The model under review builds one solid part; all positions refer to its coordinate system, in mm. A direction names the side the tool comes from. Coordinates: 2 decimals unless noted, no trailing zeros. Write each loop counter-clockwise with the first axis right and the second up, starting at its lowest first coordinate (ties: lowest second). Pieces come first, ordered by that corner, then holes.
1) Add section B-B, the plane y = -1.65. State the section outline as (x, z) points.
2) Add section C-C, the plane y = 0. State the section outline as (x, z) points.
3) Machinability: for faces 1 (the cylindrical face through (0.945, 0.724, 0.178)), 2 (the cylindrical face through (2.46, -0.11, 12.99)), which of the approach directions +Z, -Z, +X, -X, +Y, -Y give a long, thin tool a straight path to every point of the face, cutting with its end or side? Answer none if there is none.
4) Mouldability with a two-part tool opening along Z and no side actions: class faces 3 (the flat face through (-1, -1, -12.7)), 4 (the cylindrical face through (2.46, -0.11, -12.98)), 5 (the flat face through (1, -1, 12.7)) as released by +Z, released by -Z, zero draft, split by the parting line, or undercut.
5) For P1, Ø1.5, axis at x = 0, y = -1, coming from the -Z side; P2, Ø1, axis at x = -0.5, y = -1, coming from the +Z side; P3, Ø1.5, axis at x = 1, y = -2, coming from the +Z side, all flat-tipped, find the tip position at first contact; note any pin that passes through.
6) Add section D-D, the plane x = 0.7. State the section outline as (y, z) points, then the cut area to 3 significant figures.
7) Add section A-A, the plane x = -1.5. State the section outline as (y, z) points, then the cut area to 3 significant figures.
8) For line 1 (Z direction, x = -1.3, y = 2); line 2 (Z direction, x = 0.65, y = -1.55); line 3 (X direction, y = 0.5, z = -2.75), list the stretches that pass through material, from the lowest coordinate up.
from build123d import *
from OCP.BRepFilletAPI import BRepFilletAPI_MakeChamfer

# Parameters (mm, degrees)
SKETCH1_R           = 1.190625
EXTRUDE1_DEPTH      = 12.7
SKETCH1_W           = 9.8552
SKETCH1_H           = 1.27
EXTRUDE1_2_DEPTH    = 12.7
SKETCH20_R          = 1.4224
EXTRUDE24_DEPTH     = 20.045522232
CHAMFER2_SIZE       = 0.635
CHAMFER2_SIZE2      = 0.551997079
EXTRUDE4_DEPTH      = 19.94700397
EXTRUDE4_DEPTH_BACK = 19.94700397
SKETCH8_W           = 5.6896
SKETCH8_H           = 8.466666666
SKETCH9_R           = 1.190625
EXTRUDE5_DEPTH      = 8.466666667


# Read off the part's stored shape, not the designer's step: Mirror2
with BuildPart() as part:
    # Sketch1 → Extrude1 (new, symmetric)
    with BuildSketch(Plane.XY):
        with BuildLine():
            Line((12.7, -2.157017049), (1.190625, -2.157017049))
            ThreePointArc((1.190625, -2.157017049), (-1.856577095, 1.619701185), (2.298588957, -0.887017049))
            Line((2.298588957, -0.887017049), (12.7, -0.887017049))
            Line((12.7, -0.887017049), (12.7, -2.157017049))
        make_face()
        Circle(SKETCH1_R, mode=Mode.SUBTRACT)
    extrude(amount=EXTRUDE1_DEPTH, both=True)

    # Mirror2 outline → Mirror2 (revolve, cut)
    with BuildSketch(Plane(origin=(8.3312, 0, -7.8486), x_dir=(1, 0, 0), z_dir=(0, 0, 1))):
        Polygon((1.784715731, -0.887017049), (0, -0.887017049), (0, -1.93881362), (1.4224, -1.93881362), (1.4224, -1.30381362), align=None)
    revolve(axis=Axis((8.3312, 0, -7.8486), (0, 1, 0)), mode=Mode.SUBTRACT)

    # Mirror2 2 outline → Mirror2 2 (revolve, cut)
    with BuildSketch(Plane(origin=(8.3312, 0, 7.8486), x_dir=(1, 0, 0), z_dir=(0, 0, 1))):
        Polygon((0, -0.887017049), (0, -1.93881362), (1.4224, -1.93881362), (1.4224, -1.30381362), (1.784715731, -0.887017049), align=None)
    revolve(axis=Axis((8.3312, 0, 7.8486), (0, 1, 0)), mode=Mode.SUBTRACT)

    # Sketch8 → Extrude4 (cut, two sides: drawn at the far end of the back side and taken through both)
    with BuildSketch(Plane(origin=(0, 0, 0), x_dir=(1, 0, 0), z_dir=(0, 1, 0)).offset(-EXTRUDE4_DEPTH_BACK)):
        Rectangle(SKETCH8_W, SKETCH8_H)
    extrude(amount=EXTRUDE4_DEPTH + EXTRUDE4_DEPTH_BACK, mode=Mode.SUBTRACT)


with BuildPart() as body_2:
    # Sketch1 → Extrude1 2 (new, symmetric)
    with BuildSketch(Plane.XY):
        with Locations((-7.7724, -1.30381362)):
            Rectangle(SKETCH1_W, SKETCH1_H)
    extrude(amount=EXTRUDE1_2_DEPTH, both=True)

    # Sketch20 → Extrude24 (cut, through all)
    with BuildSketch(Plane(origin=(0, -0.66881362, 0), x_dir=(1, 0, 0), z_dir=(0, 1, 0))):
        with Locations(Location((-8.3312, 7.8486, 0), (0, 0, 270))):
            Circle(SKETCH20_R)
        with Locations(Location((-8.3312, -7.8486, 0), (0, 0, 270))):
            Circle(SKETCH20_R)
    extrude(amount=-EXTRUDE24_DEPTH, mode=Mode.SUBTRACT)

    # Chamfer2: one chamfer whose edges measure the first distance from different faces: ONE call of the kernel's chamfer builder (chamfer() names one face for all edges)
    chamfer2_edges_1 = [body_2.edges().sort_by_distance(p)[0] for p in [
        (-8.3312, -0.66881362, -9.271),
    ]]
    chamfer2_side_1 = [body_2.faces().sort_by_distance(p)[0] for p in [
        (-8.3312, -1.30381362, -9.271),
    ]]
    chamfer2_edges_2 = [body_2.edges().sort_by_distance(p)[0] for p in [
        (-8.3312, -0.66881362, 6.4262),
    ]]
    chamfer2_side_2 = [body_2.faces().sort_by_distance(p)[0] for p in [
        (-8.3312, -1.30381362, 6.4262),
    ]]
    chamfer2 = BRepFilletAPI_MakeChamfer(body_2.part.solid().wrapped)
    for e in chamfer2_edges_1:
        chamfer2.Add(CHAMFER2_SIZE, CHAMFER2_SIZE2, e.wrapped, chamfer2_side_1[0].wrapped)  # the first distance lies on this face
    for e in chamfer2_edges_2:
        chamfer2.Add(CHAMFER2_SIZE, CHAMFER2_SIZE2, e.wrapped, chamfer2_side_2[0].wrapped)  # the first distance lies on this face
    add(Compound.cast(chamfer2.Shape()), mode=Mode.REPLACE)

    # Sketch9 → Extrude5 (add)
    with BuildSketch(Plane.XY.offset(-4.233333333)):
        with BuildLine():
            Line((-2.371286314, -0.66881362), (-2.8448, -0.66881362))
            Line((-2.8448, -0.66881362), (-2.8448, -1.93881362))
            Line((-2.8448, -1.93881362), (-1.520300032, -1.93881362))
            ThreePointArc((-1.520300032, -1.93881362), (2.046786768, 1.371486189), (-2.371286314, -0.66881362))
        make_face()
        with Locations(Location((0, 0, 0), (0, 0, 180))):
            Circle(SKETCH9_R, mode=Mode.SUBTRACT)
    extrude(amount=EXTRUDE5_DEPTH)


with BuildPart() as body_3:
    # Sketch6 → Revolve1 (revolve)
    with BuildSketch(Plane(origin=(0, 0, 0), x_dir=(1, 0, 0), z_dir=(0, 1, 0))):
        with BuildLine():
            Line((-2.4638, -12.7), (-2.4638, -13.2715))
            ThreePointArc((-2.4638, -13.2715), (-1.264606924, -13.698253184), (0, -13.843))
            Line((0, -13.843), (0, 13.843))
            ThreePointArc((0, 13.843), (-1.264606924, 13.698253184), (-2.4638, 13.2715))
            Line((-2.4638, 13.2715), (-2.4638, 12.7))
            Line((-2.4638, 12.7), (-1.190625, 12.7))
            Line((-1.190625, 12.7), (-1.190625, -12.7))
            Line((-1.190625, -12.7), (-2.4638, -12.7))
        make_face()
    revolve(axis=Axis((0, 0, -13.843), (0, 0, 1)))


solid = body_3.part
Geometry results:
1. outline: (-1.83, -13.27) arc R5.35 ccw to (1.83, -13.27) - (1.83, -12.7) - (-1.83, -12.7) - close; (-1.83, 12.7) - (1.83, 12.7) - (1.83, 13.27) arc R5.35 ccw to (-1.83, 13.27) - close
2. outline: (-2.46, -13.27) arc R5.6 ccw to (2.46, -13.27) - (2.46, -12.7) - (1.19, -12.7) - (1.19, 12.7) - (2.46, 12.7) - (2.46, 13.27) arc R5.6 ccw to (-2.46, 13.27) - (-2.46, 12.7) - (-1.19, 12.7) - (-1.19, -12.7) - (-2.46, -12.7) - close
3. face 1: none
3. face 2: +Z, -Z
4. face 3: undercut
4. face 4: zero draft
4. face 5: undercut
5. P1: stops at z = -13.84
5. P2: stops at z = 13.81
5. P3: stops at z = 13.64
6. outline: (-2.36, -13.27) arc R5.55 ccw to (2.36, -13.27) - (2.36, -12.7) - (0.96, -12.7) - (0.96, 12.7) - (2.36, 12.7) - (2.36, 13.27) arc R5.55 ccw to (-2.36, 13.27) - (-2.36, 12.7) - (-0.96, 12.7) - (-0.96, -12.7) - (-2.36, -12.7) - close
6. area: 57.7 mm2
7. outline: (-1.95, -13.27) arc R5.39 ccw to (1.95, -13.27) - (1.95, -12.7) - (-1.95, -12.7) - close; (-1.95, 12.7) - (1.95, 12.7) - (1.95, 13.27) arc R5.39 ccw to (-1.95, 13.27) - close
7. area: 6.39 mm2
8. line 1: z = -13.31 to -12.7, 12.7 to 13.31
8. line 2: z = -13.58 to -12.7, 12.7 to 13.58
8. line 3: x = -1.08 to 1.08
